```python
from build123d import *

# Parameters (mm, degrees)
F0_R     = 2
F0_R_2   = 12.5476
F0_R_3   = 2.50063
F1_DEPTH = 60.3
F2_DEPTH = 3.048
F3_DEPTH = 21.844
F4_SIZE  = 0.5


with BuildPart() as f1:
    # F0 (on Top) → F1 (new body)
    with BuildSketch(Plane.XY):
        with BuildLine():
            ThreePointArc((21.0058, 16.0058), (19.541334, 19.541334), (16.0058, 21.0058))
            Line((16.0058, 21.0058), (-16.0058, 21.0058))
            ThreePointArc((-16.0058, 21.0058), (-19.541334, 19.541334), (-21.0058, 16.0058))
            Line((-21.0058, 16.0058), (-21.0058, -16.0058))
            ThreePointArc((-21.0058, -16.0058), (-19.541334, -19.541334), (-16.0058, -21.0058))
            Line((-16.0058, -21.0058), (16.0058, -21.0058))
            ThreePointArc((16.0058, -21.0058), (19.541334, -19.541334), (21.0058, -16.0058))
            Line((21.0058, -16.0058), (21.0058, 16.0058))
        make_face()
        with Locations((-12.725023, -12.725023)):
            Circle(F0_R, mode=Mode.SUBTRACT)
        with Locations((12.725023, -12.725023)):
            Circle(F0_R, mode=Mode.SUBTRACT)
        with Locations((-12.725023, 12.725023)):
            Circle(F0_R, mode=Mode.SUBTRACT)
        Circle(F0_R_2, mode=Mode.SUBTRACT)
        with Locations((12.725023, 12.725023)):
            Circle(F0_R, mode=Mode.SUBTRACT)
        Circle(F0_R_2)
        Circle(F0_R_3, mode=Mode.SUBTRACT)
    extrude(amount=-F1_DEPTH)

    # F0 (on Top) → F2 (join)
    with BuildSketch(Plane.XY):
        Circle(F0_R_2)
        Circle(F0_R_3, mode=Mode.SUBTRACT)
    extrude(amount=F2_DEPTH)

    # F0 (on Top) → F3 (join)
    with BuildSketch(Plane.XY):
        Circle(F0_R_3)
    extrude(amount=F3_DEPTH)

    # F4
    f4_edges = [f1.edges().sort_by_distance(p)[0] for p in [
        (-2.50063, 0, 21.844),
        (-12.5476, 0, 3.048),
        (-14.725023, -12.725023, 0),
        (-14.725023, 12.725023, 0),
        (10.725023, 12.725023, 0),
        (10.725023, -12.725023, 0),
        (19.541334, 19.541334, 0),
        (21.0058, 0, 0),
        (0, 21.0058, 0),
        (19.541334, -19.541334, 0),
        (-19.541334, 19.541334, 0),
        (0, -21.0058, 0),
        (-21.0058, 0, 0),
        (-19.541334, -19.541334, 0),
        (-12.5476, 0, 0),
        (19.541334, 19.541334, -60.3),
        (0, 21.0058, -60.3),
        (-19.541334, 19.541334, -60.3),
        (-21.0058, 0, -60.3),
        (-19.541334, -19.541334, -60.3),
        (0, -21.0058, -60.3),
        (19.541334, -19.541334, -60.3),
        (21.0058, 0, -60.3),
        (-14.725023, -12.725023, -60.3),
        (10.725023, -12.725023, -60.3),
        (-14.725023, 12.725023, -60.3),
        (10.725023, 12.725023, -60.3),
        (-2.50063, 0, -60.3),
    ]]
    chamfer(f4_edges, length=F4_SIZE)


solid = f1.part
```
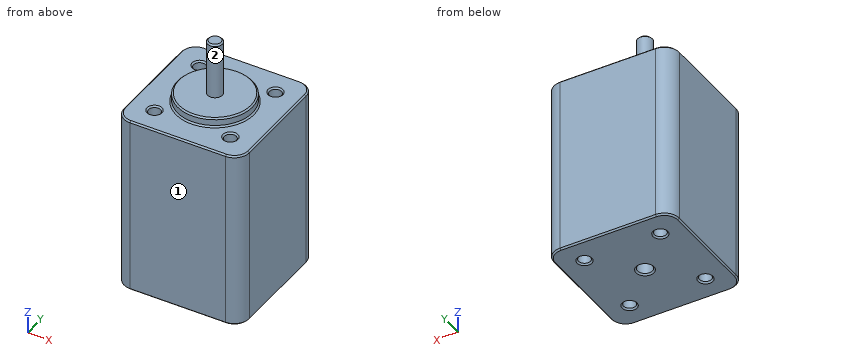
Source: CAD feature listing. Evaluate the final solid. Frame: model axes, mm. Face numbers are marked on the shaded views. A direction names the side the tool comes from. Give positions to 0.01 mm unless a question says otherwise; leave off trailing zeros. Write each loop counter-clockwise with the first axis right and the second up, starting at its lowest first coordinate (ties: lowest second). Pieces come first, ordered by that corner, then holes.
1. Section query D-D (z = 5). Return the cut outline in (x, y).
2. Material intervals for line 1 along X through (y, z) = (13, -23); line 2 along Y through (x, z) = (-13.5, -52.5); line 3 along Y through (x, z) = (0, -19), sorted ascending.
3. Section query B-B (z = -37). Return the cut outline in (x, y).
4. Access query for the marked faces 1 and 2. Directions: +Z, -Z, +X, -X, +Y, -Y. A direction counts if a zero-diameter tool reaches every point of the face in a straight line with its end or side. Return the directions, or none.
5. Section query A-A (x = 0). Return the cut outline in (y, z).
6. First-contact query: pin 1 (1 mm diameter, centred on x = -11, y = 8, fed in from +Z); pin 2 (3 mm diameter, centred on x = -12.73, y = -12.73, fed in from +Z); pin 3 (6.5 mm diameter, centred on x = -12.73, y = 12.73, fed in from -Z); pin 4 (12.5 mm diameter, centred on x = 7.5, y = -8.5, fed in from +Z). Flat tips, straight axial feed; report the tip coordinate or a pass-through.
Output values:
1. outline: circle Ø5 at (0, 0)
2. line 1: x = -21.01 to -14.71, -10.74 to 10.74, 14.71 to 21.01
2. line 2: y = -21.01 to -14.57, -10.88 to 10.88, 14.57 to 21.01
2. line 3: y = -21.01 to -2.5, 2.5 to 21.01
3. outline: (-21.01, -16.01) arc R5 ccw to (-16.01, -21.01) - (16.01, -21.01) arc R5 ccw to (21.01, -16.01) - (21.01, 16.01) arc R5 ccw to (16.01, 21.01) - (-16.01, 21.01) arc R5 ccw to (-21.01, 16.01) - close; hole circle Ø4 at (-12.73, -12.73); hole circle Ø4 at (-12.73, 12.73); hole circle Ø5 at (0, 0); hole circle Ø4 at (12.73, -12.73); hole circle Ø4 at (12.73, 12.73)
4. face 1: +Z, -Z, +X, -X, -Y
4. face 2: +Z
5. outline: (-21.01, -59.8) - (-20.51, -60.3) - (-3, -60.3) - (-2.5, -59.8) - (-2.5, 0) - (2.5, 0) - (2.5, -59.8) - (3, -60.3) - (20.51, -60.3) - (21.01, -59.8) - (21.01, -0.5) - (20.51, 0) - (13.05, 0) - (12.55, 0.5) - (12.55, 2.55) - (12.05, 3.05) - (2.5, 3.05) - (2.5, 21.34) - (2, 21.84) - (-2, 21.84) - (-2.5, 21.34) - (-2.5, 3.05) - (-12.05, 3.05) - (-12.55, 2.55) - (-12.55, 0.5) - (-13.05, 0) - (-20.51, 0) - (-21.01, -0.5) - close
6. pin 1: stops at z = 0
6. pin 2: passes through
6. pin 3: stops at z = -60.3
6. pin 4: stops at z = 3.05
